from build123d import *

# Parameters (mm, degrees)
BOSS_EXTRUDE1_DEPTH                                 = 150
CBORE_FOR_M4_HEX_SOCKET_HEAD_CAP_SCREW1_D           = 4.5
CBORE_FOR_M4_HEX_SOCKET_HEAD_CAP_SCREW1_CBORE_D     = 8
CBORE_FOR_M4_HEX_SOCKET_HEAD_CAP_SCREW1_CBORE_DEPTH = 4.4
MIRROR3_COPY_1_D                                    = 4.5
MIRROR3_COPY_1_CBORE_D                              = 8
MIRROR3_COPY_1_CBORE_DEPTH                          = 4.4
CBORE_FOR_M6_HEX_SOCKET_HEAD_CAP_SCREW1_D           = 6.6
CBORE_FOR_M6_HEX_SOCKET_HEAD_CAP_SCREW1_DEPTH       = 23.63
CBORE_FOR_M6_HEX_SOCKET_HEAD_CAP_SCREW1_CBORE_D     = 11
CBORE_FOR_M6_HEX_SOCKET_HEAD_CAP_SCREW1_CBORE_DEPTH = 6.4


with BuildPart() as part:
    # Sketch1 → Boss-Extrude1 (new body)
    with BuildSketch(Plane.XY):
        Polygon((-37.5, 0), (37.5, 0), (37.5, -14.13), (77.5, -14.13), (77.5, 0), (85, 0), (85, 9.5), (-85, 9.5), (-85, 0), (-77.5, 0), (-77.5, -14.13), (-37.5, -14.13), align=None)
    extrude(amount=BOSS_EXTRUDE1_DEPTH)

    # CBORE for M4 Hex Socket Head Cap Screw1 (through all)
    with Locations(Plane(origin=(-5.289478712, 9.5, 140.046555309), x_dir=(1, 0, 0), z_dir=(0, 1, 0))):
        with Locations((75.789478712, 31.196555309), (49.789478712, 5.196555309), (49.789478712, 31.196555309), (75.789478712, 5.196555309)):
            cbore_for_m4_hex_socket_head_cap_screw1 = CounterBoreHole(CBORE_FOR_M4_HEX_SOCKET_HEAD_CAP_SCREW1_D / 2, CBORE_FOR_M4_HEX_SOCKET_HEAD_CAP_SCREW1_CBORE_D / 2, CBORE_FOR_M4_HEX_SOCKET_HEAD_CAP_SCREW1_CBORE_DEPTH)

    # Mirror2: CBORE for M4 Hex Socket Head Cap Screw1 across plane
    add(cbore_for_m4_hex_socket_head_cap_screw1.mirror(Plane(origin=(0, 0, 0), x_dir=(0, 0, 1), z_dir=(1, 0, 0))), mode=Mode.SUBTRACT)

    # Mirror3: CBORE for M4 Hex Socket Head Cap Screw1 across plane
    add(cbore_for_m4_hex_socket_head_cap_screw1.mirror(Plane.XY.offset(75)), mode=Mode.SUBTRACT)

    # Mirror3 copy 1 (through all)
    with Locations(Plane(origin=(5.289478712, 9.5, 9.953444691), x_dir=(-1, 0, 0), z_dir=(0, 1, 0))):
        with Locations((75.789478712, 31.196555309), (49.789478712, 5.196555309), (49.789478712, 31.196555309), (75.789478712, 5.196555309)):
            CounterBoreHole(MIRROR3_COPY_1_D / 2, MIRROR3_COPY_1_CBORE_D / 2, MIRROR3_COPY_1_CBORE_DEPTH)

    # CBORE for M6 Hex Socket Head Cap Screw1
    with Locations(Plane(origin=(-5.289478712, 9.5, 140.046555309), x_dir=(1, 0, 0), z_dir=(0, 1, 0))):
        with Locations((27.789478712, 0.046555309), (-17.210521288, 0.046555309)):
            CounterBoreHole(CBORE_FOR_M6_HEX_SOCKET_HEAD_CAP_SCREW1_D / 2, CBORE_FOR_M6_HEX_SOCKET_HEAD_CAP_SCREW1_CBORE_D / 2, CBORE_FOR_M6_HEX_SOCKET_HEAD_CAP_SCREW1_CBORE_DEPTH, depth=CBORE_FOR_M6_HEX_SOCKET_HEAD_CAP_SCREW1_DEPTH)


solid = part.part
Verification items for the finished model (mm, model axes). A direction names the side the tool comes from. Coordinates: 2 decimals unless noted, no trailing zeros. Order: outer loops, then holes, each group sorted by start corner. A loop starts at its lowest first (then second) coordinate and runs counter-clockwise, first axis right, second up. Notation, with made-up numbers: M 76,52 L 94,52 A19 ccw 94,78 Z; hole C 33,-38 d8. An arc over 180 degrees is marked long. One line per item, written item: value. Start each with the question number.
Item 1: Mould release check, pull along X, two halves, no side actions. Record for faces 3 (the cylindrical face through (23.22, 1.53, 143.22)), 4 (the flat face through (85, 5, 74)), 5 (the flat face through (81, 0, 74)): released by +X, released by -X, zero draft, split by the parting line, or undercut.
Item 2: Gauge pin test, flat ends, axial feed: pin 1 (4 mm diameter, centred on y = -4, z = 57, fed in from +X); pin 2 (8 mm diameter, centred on x = 25, z = 134, fed in from -Y); pin 3 (5.5 mm diameter, centred on x = 22.5, z = 140, fed in from -Y). Record the tip position at first contact, or that the pin passes through.
Item 3: Scan lines: probe 1 along Z at (x, y) = (-44.5, -2); probe 2 along Z at (x, y) = (44.5, 6.85); probe 3 along X at (y, z) = (-8, 30). Record each from-to range of solid material in increasing order.
Item 4: Sectioned sample at B-B (x = -22.5). Enter the section's corners in (y, z).
Item 5: Access from +Z, -Z, +X, -X, +Y, -Y to the whole of each face (thin tool, end or side, straight path). Record for faces 1 (the flat face through (-46, 5.1, 13)), 2 (the cylindrical face through (-21.78, 1.53, 143.22)).
Item 6: Sectioned sample at C-C (z = 82). Enter the section's corners in (x, y), then the cut area to 3 significant figures.
Item 7: Sectioned sample at A-A (y = -3.25). Count the separate pieces of the cut face and the enclosed holes in it, then the cut area to 3 significant figures.
Conclusion:
1. face 3: undercut
1. face 4: released by +X
1. face 5: zero draft
2. pin 1: stops at x = 77.5
2. pin 2: stops at y = 0
2. pin 3: passes through
3. probe 1: z = 0 to 12.9, 17.4 to 38.9, 43.4 to 106.6, 111.1 to 132.6, 137.1 to 150
3. probe 2: z = 0 to 11.15, 19.15 to 37.15, 45.15 to 104.85, 112.85 to 130.85, 138.85 to 150
3. probe 3: x = -77.5 to -37.5, 37.5 to 77.5
4. outline: M 0,0 L 9.5,0 L 9.5,134.5 L 3.1,134.5 L 3.1,136.7 L 0,136.7 Z; M 0,143.3 L 3.1,143.3 L 3.1,145.5 L 9.5,145.5 L 9.5,150 L 0,150 Z
5. face 1: +Y
5. face 2: +Y, -Y
6. outline: M -85,0 L -77.5,0 L -77.5,-14.13 L -37.5,-14.13 L -37.5,0 L 37.5,0 L 37.5,-14.13 L 77.5,-14.13 L 77.5,0 L 85,0 L 85,9.5 L -85,9.5 Z
6. area: 2,750 mm^2
7. separate pieces: 2
7. enclosed holes: 16
7. area: 11,700 mm^2
